```python
from build123d import *

# Parameters (mm, degrees)
BOSS_EXTRUDE2_DEPTH = 2.54


with BuildPart() as part:
    # Sketch1 → Boss-Extrude2 (new body)
    with BuildSketch(Plane.XY):
        Polygon((280.770009641, 372.365015451), (280.770009641, 169.165015451), (242.670009641, 169.165015451), (39.470009641, 169.165015451), (1.370009641, 169.165015451), (1.370009641, 372.365015451), align=None)
        Polygon((280.770009641, 372.365015451), (747.609563641, 372.365015451), (747.609563641, 524.765015451), (280.770009641, 524.765015451), (-24.029990359, 524.765015451), (-465.469544359, 524.765015451), (-465.469544359, 372.365015451), (1.370009641, 372.365015451), align=None)
        with BuildLine():
            Line((1.370009641, 372.365015451), (1.370009641, 169.165015451))
            Line((1.370009641, 169.165015451), (39.470009641, 123.208075057))
            Line((39.470009641, 123.208075057), (39.470009641, -195.172287059))
            Line((39.470009641, -195.172287059), (-155.062591517, 39.476614679))
            ThreePointArc((-155.062591517, 39.476614679), (-182.536111841, 255.58711032), (1.370009641, 372.365015451))
        make_face()
        with BuildLine():
            ThreePointArc((280.770009641, 372.365015451), (464.676131123, 255.58711032), (437.202610799, 39.476614679))
            Line((437.202610799, 39.476614679), (242.670009641, -195.172287059))
            Line((242.670009641, -195.172287059), (242.670009641, 123.208075057))
            Line((242.670009641, 123.208075057), (280.770009641, 169.165015451))
            Line((280.770009641, 169.165015451), (280.770009641, 372.365015451))
        make_face()
        Polygon((554.527061668, -57.7896859), (457.260761089, -175.114136769), (242.670009641, -195.172287059), (437.202610799, 39.476614679), align=None)
        Polygon((-272.387042386, -57.7896859), (-155.062591517, 39.476614679), (39.470009641, -195.172287059), (-175.120741807, -175.114136769), align=None)
    extrude(amount=BOSS_EXTRUDE2_DEPTH)


solid = part.part
```
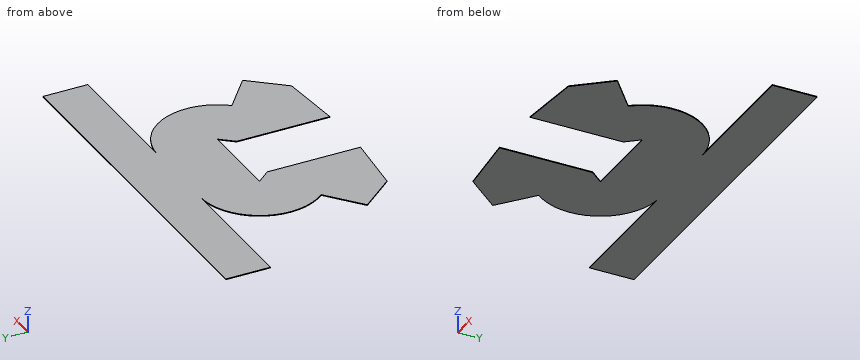
Input: part model. Units: mm. Frame: model coordinates. Give positions to 0.01 mm unless a question says otherwise; leave off trailing zeros. Order: outer loops, then holes, each group sorted by start corner. A loop starts at its lowest first (then second) coordinate and runs counter-clockwise, first axis right, second up. Notation, with made-up numbers: M 14.25,-3.75 L 68.25,-3.75 A11 ccw 68.25,3.25 Z; hole C 37,11 d10. An arc over 180 degrees is marked long. One line per question, with ' | ' between items. Start each with the question number.
1. First-contact query: pin 1 Ø1 at (x, z) = (506.5, 1.5) entering from -Y; pin 2 Ø0.8 at (x, z) = (88, 1.5) entering from -Y (3 decimals). Flat tips, straight axial feed; report the tip coordinate or a pass-through.
2. Section query B-B (z = 1.75). Return the cut outline in (x, y).
3. Section query D-D (y = 206.5). Return the cut outline in (x, z), and give its area (3 significant figures).
4. Section query C-C (x = 342). Return the cut outline in (y, z).
5. Section query A-A (x = -39.5). Return the cut outline in (y, z).
6. Material intervals for probe 1 along Y at (x, z) = (162.5, 2.05); probe 2 along X at (y, z) = (-11, 1.85); probe 3 along X at (y, z) = (-79.5, 1.3), sorted ascending. Write a range as [from, to].
Here are the results:
1) pin 1: y = -116.32 | pin 2: y = 169.165
2) outline: M -465.47,372.37 L 1.37,372.37 A203.2 ccw -155.06,39.48 L -272.39,-57.79 L -175.12,-175.11 L 39.47,-195.17 L 39.47,123.21 L 1.37,169.17 L 280.77,169.17 L 242.67,123.21 L 242.67,-195.17 L 457.26,-175.11 L 554.53,-57.79 L 437.2,39.48 A203.2 ccw 280.77,372.37 L 747.61,372.37 L 747.61,524.77 L -465.47,524.77 Z
3) outline: M -198.37,0 L 480.51,0 L 480.51,2.54 L -198.37,2.54 Z | area: 1,720 mm²
4) outline: M -185.89,0 L 362.92,0 L 362.92,2.54 L -185.89,2.54 Z; M 372.37,0 L 524.77,0 L 524.77,2.54 L 372.37,2.54 Z
5) outline: M -187.79,0 L 368.21,0 L 368.21,2.54 L -187.79,2.54 Z; M 372.37,0 L 524.77,0 L 524.77,2.54 L 372.37,2.54 Z
6) probe 1: [169.17, 524.77] | probe 2: [-215.95, 39.47], [242.67, 498.09] | probe 3: [-254.39, 39.47], [242.67, 536.53]
